Input: part model. Units: mm. Frame: model coordinates. Round coordinates to 2 decimals unless told otherwise and drop trailing zeros. Write each loop counter-clockwise with the first axis right and the second up, starting at its lowest first coordinate (ties: lowest second). Pieces come first, ordered by that corner, then holes. Notation, with made-up numbers: (3.25, 60.5) -> (24.25, 60.5) arc R17 cw to (24.25, 80.5) -> close; hole circle Ø9 at (-7.5, 79). An arc over 180 degrees is marked (long way). Write item = value, one per line.
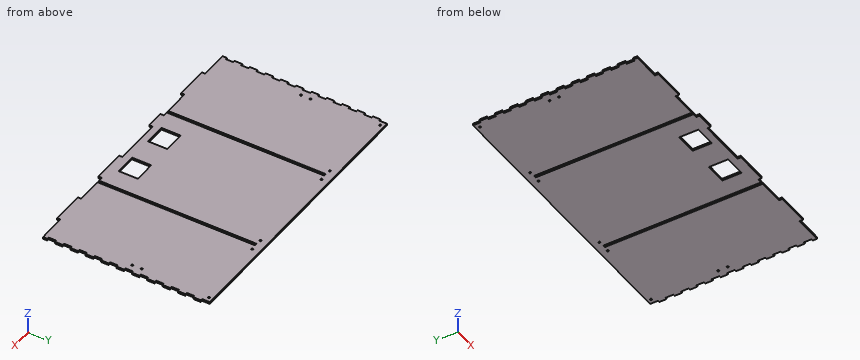
```python
from build123d import *

# Parameters (mm, degrees)
SKETCH1_W                    = 3.175
SKETCH1_H                    = 12.7
MAIN_EXTRUDE_DEPTH           = 3.175
SKETCH8_R                    = 1.5
SKETCH8_W                    = 3.175
SKETCH8_H                    = 31.877
MOUNT_HOLES_DEPTH            = 4.175
SKETCH3_W                    = 4
SKETCH3_H                    = 260.604
DOOR_SLOTS_DEPTH             = 10
SKETCH10_R                   = 1.5
DOOR_GUIDE_MOUNT_HOLES_DEPTH = 4.175
SKETCH12_R                   = 1.5
EXTENSION_CLIP_HOLES_DEPTH   = 4.175
EXTENSION_CENTER_CUT_DEPTH   = 4.175
SKETCH17_W                   = 35
SKETCH17_H                   = 31.75
SKETCH17_W_2                 = 24.976666667
SKETCH17_H_2                 = 5.588
NOSEPOKEHOLES_DEPTH          = 10


with BuildPart() as part:
    # Sketch1 → Main Extrude (new body)
    with BuildSketch(Plane.XY):
        Polygon((-243.84, -134.112), (-189.653333333, -134.112), (-189.653333333, -139.7), (-135.466666667, -139.7), (-135.466666667, -134.112), (-81.28, -134.112), (-81.28, -139.7), (-27.093333333, -139.7), (-27.093333333, -134.112), (27.093333333, -134.112), (27.093333333, -139.7), (81.28, -139.7), (81.28, -134.112), (135.466666667, -134.112), (135.466666667, -139.7), (189.653333333, -139.7), (189.653333333, -134.112), (243.84, -134.112), (243.84, -139.7), (298.026666667, -139.7), (298.026666667, -134.112), (352.213333333, -134.112), (352.213333333, -139.7), (406.4, -139.7), (406.4, 139.7), (381, 139.7), (381, 127), (377.825, 127), (377.825, 139.7), (-377.825, 139.7), (-377.825, 127), (-381, 127), (-381, 139.7), (-406.4, 139.7), (-406.4, -139.7), (-352.213333333, -139.7), (-352.213333333, -134.112), (-298.026666667, -134.112), (-298.026666667, -139.7), (-243.84, -139.7), align=None)
        with Locations((-379.4125, -120.65)):
            Rectangle(SKETCH1_W, SKETCH1_H, mode=Mode.SUBTRACT)
        with Locations((-379.4125, -95.25)):
            Rectangle(SKETCH1_W, SKETCH1_H, mode=Mode.SUBTRACT)
        with Locations((379.4125, 82.55)):
            Rectangle(SKETCH1_W, SKETCH1_H, mode=Mode.SUBTRACT)
        with Locations((379.4125, 57.15)):
            Rectangle(SKETCH1_W, SKETCH1_H, mode=Mode.SUBTRACT)
        with Locations((379.4125, 31.75)):
            Rectangle(SKETCH1_W, SKETCH1_H, mode=Mode.SUBTRACT)
        with Locations((379.4125, 6.35)):
            Rectangle(SKETCH1_W, SKETCH1_H, mode=Mode.SUBTRACT)
        with Locations((379.4125, -19.05)):
            Rectangle(SKETCH1_W, SKETCH1_H, mode=Mode.SUBTRACT)
        with Locations((379.4125, -44.45)):
            Rectangle(SKETCH1_W, SKETCH1_H, mode=Mode.SUBTRACT)
        with Locations((379.4125, -69.85)):
            Rectangle(SKETCH1_W, SKETCH1_H, mode=Mode.SUBTRACT)
        with Locations((379.4125, -95.25)):
            Rectangle(SKETCH1_W, SKETCH1_H, mode=Mode.SUBTRACT)
        with Locations((379.4125, -120.65)):
            Rectangle(SKETCH1_W, SKETCH1_H, mode=Mode.SUBTRACT)
        with Locations((-379.4125, -69.85)):
            Rectangle(SKETCH1_W, SKETCH1_H, mode=Mode.SUBTRACT)
        with Locations((-379.4125, -44.45)):
            Rectangle(SKETCH1_W, SKETCH1_H, mode=Mode.SUBTRACT)
        with Locations((-379.4125, -19.05)):
            Rectangle(SKETCH1_W, SKETCH1_H, mode=Mode.SUBTRACT)
        with Locations((-379.4125, 6.35)):
            Rectangle(SKETCH1_W, SKETCH1_H, mode=Mode.SUBTRACT)
        with Locations((-379.4125, 31.75)):
            Rectangle(SKETCH1_W, SKETCH1_H, mode=Mode.SUBTRACT)
        with Locations((-379.4125, 57.15)):
            Rectangle(SKETCH1_W, SKETCH1_H, mode=Mode.SUBTRACT)
        with Locations((-379.4125, 82.55)):
            Rectangle(SKETCH1_W, SKETCH1_H, mode=Mode.SUBTRACT)
        with Locations((-379.4125, 107.95)):
            Rectangle(SKETCH1_W, SKETCH1_H, mode=Mode.SUBTRACT)
        with Locations((379.4125, 107.95)):
            Rectangle(SKETCH1_W, SKETCH1_H, mode=Mode.SUBTRACT)
    extrude(amount=MAIN_EXTRUDE_DEPTH)

    # Sketch8 → Mount Holes (cut, through all)
    with BuildSketch(Plane.XY.offset(3.175)):
        with Locations((-393.7, -120.65)):
            Circle(SKETCH8_R)
        with Locations((393.7, -120.65)):
            Circle(SKETCH8_R)
        with Locations((-382.5875, 12.319)):
            Rectangle(SKETCH8_W, SKETCH8_H)
        with Locations((382.5875, 12.319)):
            Rectangle(SKETCH8_W, SKETCH8_H)
    extrude(amount=-MOUNT_HOLES_DEPTH, mode=Mode.SUBTRACT)

    # Sketch3 → Door Slots (cut)
    with BuildSketch(Plane.XY.offset(3.175)):
        with Locations((-90.678, -3.81)):
            Rectangle(SKETCH3_W, SKETCH3_H)
        with Locations((90.678, -3.81)):
            Rectangle(SKETCH3_W, SKETCH3_H)
    extrude(amount=-DOOR_SLOTS_DEPTH, mode=Mode.SUBTRACT)

    # Sketch10 → Door Guide Mount Holes (cut, through all)
    with BuildSketch(Plane.XY.offset(3.175)):
        with Locations((-101.678, 127.492)):
            Circle(SKETCH10_R)
        with Locations((-79.678, 127.492)):
            Circle(SKETCH10_R)
        with Locations((79.678, 127.492)):
            Circle(SKETCH10_R)
        with Locations((101.678, 127.492)):
            Circle(SKETCH10_R)
    extrude(amount=-DOOR_GUIDE_MOUNT_HOLES_DEPTH, mode=Mode.SUBTRACT)

    # Sketch12 → Extension Clip Holes (cut, through all)
    with BuildSketch(Plane.XY.offset(3.175)):
        with Locations((-246.507, 20.193)):
            Circle(SKETCH12_R)
        with Locations((-246.507, 4.445)):
            Circle(SKETCH12_R)
        with Locations((-221.107, 4.445)):
            Circle(SKETCH12_R)
        with Locations((-221.107, 20.193)):
            Circle(SKETCH12_R)
        with Locations((-243.332, 133.35)):
            Circle(SKETCH12_R)
        with Locations((-224.282, 133.35)):
            Circle(SKETCH12_R)
        with Locations((224.282, 133.35)):
            Circle(SKETCH12_R)
        with Locations((243.332, 133.35)):
            Circle(SKETCH12_R)
        with Locations((221.107, 20.193)):
            Circle(SKETCH12_R)
        with Locations((221.107, 4.445)):
            Circle(SKETCH12_R)
        with Locations((246.507, 4.445)):
            Circle(SKETCH12_R)
        with Locations((246.507, 20.193)):
            Circle(SKETCH12_R)
    extrude(amount=-EXTENSION_CLIP_HOLES_DEPTH, mode=Mode.SUBTRACT)

    # Sketch11_3 → Extension Center Cut (cut, through all)
    with BuildSketch(Plane.XY.offset(3.175)):
        Polygon((-232.2195, 127), (-232.2195, 139.7), (-406.4, 139.7), (-406.4, -139.7), (-235.3945, -139.7), (-235.3945, -127), (-232.2195, -127), (-232.2195, -114.3), (-235.3945, -114.3), (-235.3945, -101.6), (-232.2195, -101.6), (-232.2195, -88.9), (-235.3945, -88.9), (-235.3945, -76.2), (-232.2195, -76.2), (-232.2195, -63.5), (-235.3945, -63.5), (-235.3945, -50.8), (-232.2195, -50.8), (-232.2195, -38.1), (-235.3945, -38.1), (-235.3945, -25.4), (-232.2195, -25.4), (-232.2195, -12.7), (-235.3945, -12.7), (-235.3945, 0), (-232.2195, 0), (-232.2195, 12.7), (-235.3945, 12.7), (-235.3945, 25.4), (-232.2195, 25.4), (-232.2195, 38.1), (-235.3945, 38.1), (-235.3945, 50.8), (-232.2195, 50.8), (-232.2195, 63.5), (-235.3945, 63.5), (-235.3945, 76.2), (-232.2195, 76.2), (-232.2195, 88.9), (-235.3945, 88.9), (-235.3945, 101.6), (-232.2195, 101.6), (-232.2195, 114.3), (-235.3945, 114.3), (-235.3945, 127), align=None)
        Polygon((406.4, 139.7), (232.2195, 139.7), (232.2195, 127), (235.3945, 127), (235.3945, 114.3), (232.2195, 114.3), (232.2195, 101.6), (235.3945, 101.6), (235.3945, 88.9), (232.2195, 88.9), (232.2195, 76.2), (235.3945, 76.2), (235.3945, 63.5), (232.2195, 63.5), (232.2195, 50.8), (235.3945, 50.8), (235.3945, 38.1), (232.2195, 38.1), (232.2195, 25.4), (235.3945, 25.4), (235.3945, 12.7), (232.2195, 12.7), (232.2195, 0), (235.3945, 0), (235.3945, -12.7), (232.2195, -12.7), (232.2195, -25.4), (235.3945, -25.4), (235.3945, -38.1), (232.2195, -38.1), (232.2195, -50.8), (235.3945, -50.8), (235.3945, -63.5), (232.2195, -63.5), (232.2195, -76.2), (235.3945, -76.2), (235.3945, -88.9), (232.2195, -88.9), (232.2195, -101.6), (235.3945, -101.6), (235.3945, -114.3), (232.2195, -114.3), (232.2195, -127), (235.3945, -127), (235.3945, -139.7), (406.4, -139.7), align=None)
    extrude(amount=-EXTENSION_CENTER_CUT_DEPTH, mode=Mode.SUBTRACT)

    # Sketch17 → Nosepokeholes (cut)
    with BuildSketch(Plane.XY.offset(3.175)):
        with Locations((38.678, -106.237)):
            Rectangle(SKETCH17_W, SKETCH17_H)
        with Locations((-38.678, -106.237)):
            Rectangle(SKETCH17_W, SKETCH17_H)
        with Locations((-39.581666666, -136.906)):
            Rectangle(SKETCH17_W_2, SKETCH17_H_2)
    extrude(amount=-NOSEPOKEHOLES_DEPTH, mode=Mode.SUBTRACT)


solid = part.part
```
1) Cut plane A-A (x = 200). Return the cut outline in (y, z) (3 decimals), and give its area (3 significant figures).
Solutions:
outline = (-134.112, 0) -> (139.7, 0) -> (139.7, 3.175) -> (-134.112, 3.175) -> close
area = 869 mm^2
2) First-contact query: P1, Ø1.6, axis at y = -136, z = 2.5, coming from the -X side; P2, Ø1.5, axis at y = 10, z = 3, coming from the +X side; P3, Ø1.6, axis at x = -233.5, z = 1, coming from the -Y side. Flat tips, straight axial feed; report the tip coordinate or a pass-through.
Solutions:
P1 = -189.65
P2 = 232.22
P3 = -134.11
3) Cut plane B-B (z = 1). Count the separate pieces of the cut face and the enclosed holes in it, and give its area (3 significant figures).
Solutions:
separate_pieces = 1
enclosed_holes = 12
area = 125,000 mm^2
4) Line query: L1, parallel to X at y = 89.5, z = 3.05; L2, parallel to X at y = 114, z = 1; L3, parallel to X at y = 4, z = 1.45. Output: solid intervals per line, ascending. Write a range as from..to.
Solutions:
L1 = -235.39..-92.68, -88.68..88.68, 92.68..235.39
L2 = -232.22..-92.68, -88.68..88.68, 92.68..232.22
L3 = -232.22..-222.54, -219.67..-92.68, -88.68..88.68, 92.68..219.67, 222.54..232.22
